from build123d import *

# Parameters (mm, degrees)
RACCORDO1_R                    = 5
FORO_1_0_16_1_D                = 16
RIPETIZIONECIRCOLARE1_COUNT    = 6
FORO_FILETTATO_M10X1_5_1_D     = 8.5
FORO_FILETTATO_M10X1_5_1_DEPTH = 18
FORO_FILETTATO_M10X1_5_1_TIP   = 2.553657631


with BuildPart() as part:
    # Schizzo1 → Rivoluzione1 (revolve)
    with BuildSketch(Plane.XY, mode=Mode.PRIVATE) as rivoluzione1_sk:
        Polygon((0, 0), (51, 0), (51, -5), (103, -5), (103, -21), (54, -21), (54, -31), (44, -31), (22, -141), (0, -141), align=None)
    revolve(rivoluzione1_sk.sketch.rotate(Axis((0, -141, 0), (0, 1, 0)), 90), axis=Axis((0, -141, 0), (0, 1, 0)))

    # Schizzo2 → Taglia-Rivoluzione1 (revolve, cut)
    with BuildSketch(Plane.XY, mode=Mode.PRIVATE) as taglia_rivoluzione1_sk:
        Polygon((0, -141), (-11.75, -141), (-11.75, -103), (-16, -100.240017729), (-16, -86.247037966), (-11, -83), (-11, -51.143483525), (-22, -44), (-22, 0), (0, 0), align=None)
    revolve(taglia_rivoluzione1_sk.sketch.rotate(Axis((0, 0, 0), (0, -1, 0)), 270), axis=Axis((0, 0, 0), (0, -1, 0)), mode=Mode.SUBTRACT)

    # Raccordo1
    raccordo1_edges = [part.edges().sort_by_distance(p)[0] for p in [
        (0, -31, 44),
    ]]
    fillet(raccordo1_edges, radius=RACCORDO1_R)

    # Foro Ø1.0 (16)-1 (through all)
    with Locations(Plane(origin=(0, -5, 0), x_dir=(1, 0, 0), z_dir=(0, 1, 0))):
        with Locations((-76, 0)):
            foro_1_0_16_1 = Hole(FORO_1_0_16_1_D / 2)

    # RipetizioneCircolare1: Foro Ø1.0 (16)-1 ×6 about axis
    ripetizionecircolare1_axis = Axis((0, 0, 0), (0, 1, 0))
    for i in range(1, RIPETIZIONECIRCOLARE1_COUNT):
        add(foro_1_0_16_1.rotate(ripetizionecircolare1_axis, i * 360 / RIPETIZIONECIRCOLARE1_COUNT), mode=Mode.SUBTRACT)

    # Foro filettato M10x1.5-1
    with Locations(Plane(origin=(0, 0, 0), x_dir=(1, 0, 0), z_dir=(0, 1, 0))):
        with Locations((38, 0), (-38, 0)):
            Hole(FORO_FILETTATO_M10X1_5_1_D / 2, depth=FORO_FILETTATO_M10X1_5_1_DEPTH)
            with Locations((0, 0, -(FORO_FILETTATO_M10X1_5_1_DEPTH + FORO_FILETTATO_M10X1_5_1_TIP / 2))):  # 118° drill point
                Cone(0, FORO_FILETTATO_M10X1_5_1_D / 2, FORO_FILETTATO_M10X1_5_1_TIP, mode=Mode.SUBTRACT)


solid = part.part
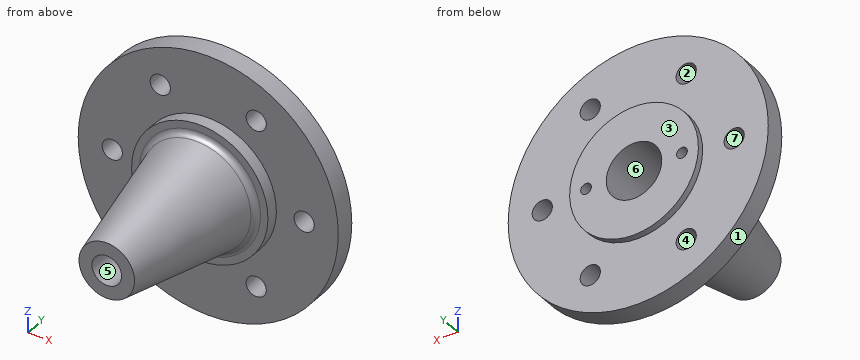
Can you work these out from the model? Positions are in its coordinate system, mm. Face numbers are marked on the shaded views. A direction names the side the tool comes from. Round coordinates to 2 decimals unless told otherwise and drop trailing zeros. Loops run counter-clockwise (first coordinate to the right, second up) from the corner with the lowest first, then second, coordinate; pieces in that order, holes last. Notation, with made-up numbers: (84.25, -11.75) - (116.25, -11.75) arc R18 cw to (116.25, 1.25) - close; hole circle Ø9 at (36, -3). An arc over 180 degrees is marked (long way). Use CSV: the item, a comma, the result in double quotes. Start each with the question number.
1) For pin 1 Ø4 at (y, z) = (-62, 25) entering from -X; pin 2 Ø12 at (y, z) = (-64, 16.5) entering from +X; pin 3 Ø9.5 at (x, z) = (38, 65.82) entering from -Y; pin 4 Ø12 at (x, z) = (62.5, 22.5) entering from -Y, each with a flat end and sliding along its axis, tell me the tip position at first contact or that it passes through.
2) If we section it at B-B on z = 69: Write out the boundary of the cut face in (x, y), plus the area to 3 significant figures.
3) For the marked faces 5, 6 and 7, which set-ups out of +Z, -Z, +X, -X, +Y, -Y let a thin tool reach every point of the face, with its end or its side?
4) If we section it at A-A on x = 76: Write out the boundary of the cut face in (y, z).
5) If we section it at D-D on x = -77: Write out the boundary of the cut face in (y, z).
6) If we section it at C-C on y = -132: Write out the boundary of the cut face in (x, z).
7) Please list where these lines run through material, in increasing order: probe 1 along Z at (x, y) = (38, -13.5); probe 2 along Y at (x, z) = (-30, 69); probe 3 along Z at (x, y) = (-7.5, -13). Write a range as [from, to].
8) We'd pull the mould along Z, two halves only. Please class the marked faces 1, 2, 3 and 4: released by +Z, released by -Z, zero draft, split by the parting line, or undercut.
Geometry results:
1,pin 1,"stops at x = -30.08"
1,pin 2,"stops at x = 36.28"
1,pin 3,"passes through"
1,pin 4,"stops at y = -21"
2,outline,"(-76.47, -21) - (-45.34, -21) - (-45.34, -5) - (-76.47, -5) - close; (-30.66, -21) - (30.66, -21) - (30.66, -5) - (-30.66, -5) - close; (45.34, -21) - (76.47, -21) - (76.47, -5) - (45.34, -5) - close"
2,area,"1,980 mm2"
3,face 5,"-Y"
3,face 6,"+Y"
3,face 7,"+Y, -Y"
4,outline,"(-21, -69.52) - (-5, -69.52) - (-5, -8) - (-21, -8) - close; (-21, 8) - (-5, 8) - (-5, 69.52) - (-21, 69.52) - close"
5,outline,"(-21, -68.41) - (-5, -68.41) - (-5, -7.94) - (-21, -7.94) - close; (-21, 7.94) - (-5, 7.94) - (-5, 68.41) - (-21, 68.41) - close"
6,outline,"circle Ø47.6 at (0, 0); hole circle Ø23.5 at (0, 0)"
7,probe 1,"z = [-95.73, -73.82], [-57.82, -4.25], [4.25, 57.82], [73.82, 95.73]"
7,probe 2,"y = [-21, -5]"
7,probe 3,"z = [-102.73, -20.68], [20.68, 102.73]"
8,face 1,"split by the parting line"
8,face 2,"undercut"
8,face 3,"zero draft"
8,face 4,"undercut"
